Could you check a few things on this model? Use its own coordinates, in mm. Face numbers are marked on the shaded views. A direction names the side the tool comes from. Give positions to 0.01 mm unless a question says otherwise; leave off trailing zeros. Loops run counter-clockwise (first coordinate to the right, second up) from the corner with the lowest first, then second, coordinate; pieces in that order, holes last. Notation, with made-up numbers: (81, 50.25) -> (117, 50.25) arc R33 cw to (117, 86.25) -> close; hole circle Ø9 at (38.25, 80.25). An arc over 180 degrees is marked (long way). Write each question's results on one line, items separated by ' | '. Start each with the question number.
Q1. If we section it at D-D, the plane z = 26.5: List the corners of the cut face in (x, y) for me.
Q2. Which directions (+Z, -Z, +X, -X, +Y, -Y) give clear straight access to the entire face, cutting with the end or side of a thin tool? Please do the marked faces 1 and 2.
Q3. If we section it at C-C, the plane y = 16: List the corners of the cut face in (x, z) for me.
Q4. We'd pull the mould along Y, two halves only. Please class the marked faces 3, 4 and 5: released by +Y, released by -Y, zero draft, split by the parting line, or undercut.
Q5. If I drill on line 1 along X through (y, z) = (52.2, 42); line 2 along Y through (x, z) = (-21.5, 39); line 3 along Z through (x, y) = (9, 43), over which ranges is the centre line in solid material (lowest first)?
Q6. If we section it at A-A, the plane y = 7.5: List the corners of the cut face in (x, z) for me.
Q7. If we section it at B-B, the plane z = 37: List the corners of the cut face in (x, y) for me, plus the area to 3 significant figures.
Q8. Will these pins go through, and if not, where does the flat tip stop? P1, Ø0.9, axis at x = 8.5, y = 39, coming from the +Z side; P2, Ø5, axis at y = 33, z = 8.5, coming from the -X side.
Autodesk Inventor part; units mm, degrees
ref_plane "YZ Plane" through (0, 0, 0) normal (1, 0, 0) x (0, 1, 0)
ref_plane "XZ Plane" through (0, 0, 0) normal (0, 1, 0) x (-1, 0, 0)
ref_plane "XY Plane" through (0, 0, 0) normal (0, 0, 1) x (1, 0, 0)
sketch "Szkic1" plane through (0, 0, 0) normal (0, 0, 1) x (1, 0, 0)
  line L0 (-24.1556, -3.6171) -> (-24.1556, -6.6171)
  line L1 (-24.1556, -6.6171) -> (10.8444, -6.6171)
  line L2 (10.8444, -6.6171) -> (10.8444, 53.3829)
  line L3 (7.8444, 50.3829) -> (7.8444, -3.6171)
  line L4 (7.8444, -3.6171) -> (-24.1556, -3.6171)
  line L5 (-24.1556, 53.3829) -> (-24.1556, 50.3829)
  line L6 (-24.1556, 50.3829) -> (7.8444, 50.3829)
  line L7 (-24.1556, 53.3829) -> (10.8444, 53.3829)
  point P0 (0, 0)
  dimension "d2" = 60
  dimension "d87" = 3
  dimension "d89" = 3
  dimension "d90" = 3
  dimension "d123" = 35
  dimension "d124" = 35
extrude "Wyciągnięcie proste1" add sketch "Szkic1" along normal blind 55.5
fillet "Zaokrąglenie1" radius 0.5 2 edges at (7.8444, -3.6171, 27.75) (7.8444, 50.3829, 27.75)
sketch "Szkic9" plane through (7.8444, -3.1171, 0) normal (-1, 0, 0) x (0, 0, 1)
  line L0 (42.5, 5.5) -> (0.5, 5.5)
  line L1 (0.5, 5.5) -> (0.5, 47.5)
  line L2 (0.5, 47.5) -> (42.5, 47.5)
  line L3 (42.5, 47.5) -> (42.5, 5.5)
  line L4 (0, 53) -> (55.5, 53)
  line L5 (0, 53) -> (0, 0)
  line L6 (55.5, 0) -> (0, 0)
  line L7 (55.5, 53) -> (55.5, 0)
  line L8 (37, 14) -> (37, 8) construction
  line L9 (35.5, 14) -> (35.5, 8)
  line L10 (38.5, 8) -> (38.5, 14)
  arc A0 (38.5, 14) -> (35.5, 14) centre (37, 14) ccw
  arc A1 (35.5, 8) -> (38.5, 8) centre (37, 8) ccw
  line L11 (37, 45) -> (37, 39) construction
  line L12 (35.5, 45) -> (35.5, 39)
  line L13 (38.5, 39) -> (38.5, 45)
  arc A2 (38.5, 45) -> (35.5, 45) centre (37, 45) ccw
  arc A3 (35.5, 39) -> (38.5, 39) centre (37, 39) ccw
  line L14 (6, 14) -> (6, 8) construction
  line L15 (4.5, 14) -> (4.5, 8)
  line L16 (7.5, 8) -> (7.5, 14)
  arc A4 (7.5, 14) -> (4.5, 14) centre (6, 14) ccw
  arc A5 (4.5, 8) -> (7.5, 8) centre (6, 8) ccw
  line L17 (6, 45) -> (6, 39) construction
  line L18 (4.5, 45) -> (4.5, 39)
  line L19 (7.5, 39) -> (7.5, 45)
  arc A6 (7.5, 45) -> (4.5, 45) centre (6, 45) ccw
  arc A7 (4.5, 39) -> (7.5, 39) centre (6, 39) ccw
  line L20 (21.5, 29.5) -> (21.5, 23.5) construction
  line L21 (10.5, 29.5) -> (10.5, 23.5)
  line L22 (32.5, 23.5) -> (32.5, 29.5)
  arc A8 (32.5, 29.5) -> (10.5, 29.5) centre (21.5, 29.5) ccw
  arc A9 (10.5, 23.5) -> (32.5, 23.5) centre (21.5, 23.5) ccw
  point P0 (0, 3.1171)
  point P1 (37, 11)
  point P2 (6, 11)
  point P3 (37, 42)
  point P4 (6, 42)
  point P5 (21.5, 26.5)
  dimension "d128" = 42
  dimension "d129" = 42
  dimension "d130" = 5.5
  dimension "d131" = 0.5
  dimension "d132" = 53
  dimension "d133" = 5.5
  dimension "d134" = 5.5
  dimension "d135" = 5.5
  dimension "d136" = 5.5
  dimension "d137" = 5.5
  dimension "d138" = 5.5
  dimension "d139" = 5.5
  dimension "d140" = 5.5
  dimension "d141" = 21
  dimension "d142" = 21
  dimension "d143" = 3
  dimension "d144" = 3
  dimension "d145" = 3
  dimension "d146" = 3
  dimension "d147" = 3
  dimension "d148" = 3
  dimension "d149" = 3
  dimension "d150" = 3
  dimension "d151" = 3
  dimension "d152" = 22
extrude "Wyciągnięcie proste4" cut sketch "Szkic9" against normal blind 3 contours A0 L10 A1 L9 | A2 L13 A3 L12 | A4 L16 A5 L15 | A6 L19 A7 L18 | A8 L22 A9 L21
sketch "Szkic10" plane through (-24.1556, -6.6171, 0) normal (0, -1, 0) x (1, 0, 0)
  line L0 (0, 0) -> (35, 0)
  line L1 (35, 0) -> (35, 55.5)
  line L2 (0, 55.5) -> (35, 55.5)
  line L3 (0, 0) -> (0, 55.5)
  line L4 (32, 55.5) -> (32, 0)
  line L5 (0, 28.5) -> (32, 28.5)
  line L6 (32, 10.5) -> (32, 32.5)
  line L7 (0, 28.5) -> (32, 0)
  point P0 (24.1556, 0)
  dimension "d155" = 28.5
extrude "Wyciągnięcie proste5" cut sketch "Szkic10" against normal up to surface (60 mm away) contours L3 L7 L0
sketch "Szkic11" plane through (-24.1556, -6.6171, 55.5) normal (0, -1, 0) x (1, 0, 0)
  line L0 (0, -27) -> (32, -55.5)
  line L1 (32, -55.5) -> (35, -55.5)
  line L2 (35, -55.5) -> (35, 0)
  line L3 (0, 0) -> (35, 0)
  line L4 (0, -27) -> (0, 0)
  line L5 (31.5, -55.0547) -> (31.5, 0)
  line L6 (32, 0) -> (32, -55.5)
  point P0 (24.1556, -55.5)
  point P1 (7.75, -13.5)
  point P2 (23.75, -13.5)
  dimension "d158" = 13.5
  dimension "d159" = 13.5
  dimension "d160" = 16
  dimension "d161" = 31.5
  dimension "d162" = 7.75
hole "Otwór7" at (-16.4056, -6.6171, 42) at (-0.4056, -6.6171, 42) direction (0, 1, 0) diameter 5 end through all
chamfer "Faza5" distance 4 angle 45 2 edges at (-24.1556, -5.1171, 55.5) (-24.1556, 51.8829, 55.5)
fillet "Zaokrąglenie6" radius 3 6 edges at (-24.1556, -5.1171, 28.5) (-24.1556, 51.8829, 28.5) (-24.1556, 51.8829, 51.5) (-20.1556, 51.8829, 55.5) (-24.1556, -5.1171, 51.5) (-20.1556, -5.1171, 55.5)
sketch "Szkic12" plane through (10.8444, -6.6171, 0) normal (1, 0, 0) x (0, 0, -1)
  line L0 (-55.5, 57) -> (-0.4453, 57)
  arc A0 (-7.5, 42.5) -> (-4.5, 42.5) centre (-6, 42.5) ccw
  line L1 (-7.5, 42.5) -> (-7.5, 48.5)
  arc A1 (-4.5, 48.5) -> (-7.5, 48.5) centre (-6, 48.5) ccw
  line L2 (-4.5, 48.5) -> (-4.5, 42.5)
  arc A2 (-38.5, 42.5) -> (-35.5, 42.5) centre (-37, 42.5) ccw
  line L3 (-38.5, 42.5) -> (-38.5, 48.5)
  arc A3 (-35.5, 48.5) -> (-38.5, 48.5) centre (-37, 48.5) ccw
  line L4 (-35.5, 48.5) -> (-35.5, 42.5)
  arc A4 (-38.5, 11.5) -> (-35.5, 11.5) centre (-37, 11.5) ccw
  line L5 (-38.5, 11.5) -> (-38.5, 17.5)
  arc A5 (-35.5, 17.5) -> (-38.5, 17.5) centre (-37, 17.5) ccw
  line L6 (-35.5, 17.5) -> (-35.5, 11.5)
  arc A6 (-7.5, 11.5) -> (-4.5, 11.5) centre (-6, 11.5) ccw
  line L7 (-7.5, 11.5) -> (-7.5, 17.5)
  arc A7 (-4.5, 17.5) -> (-7.5, 17.5) centre (-6, 17.5) ccw
  line L8 (-4.5, 17.5) -> (-4.5, 11.5)
  arc A8 (-32.5, 27) -> (-10.5, 27) centre (-21.5, 27) ccw
  line L9 (-32.5, 27) -> (-32.5, 33)
  arc A9 (-10.5, 33) -> (-32.5, 33) centre (-21.5, 33) ccw
  line L10 (-10.5, 33) -> (-10.5, 27)
  line L11 (0, 0) -> (0, 60)
  line L12 (0, 60) -> (-55.5, 60)
  line L13 (-55.5, 0) -> (-55.5, 60)
  line L14 (0, 0) -> (-55.5, 0)
  line L15 (-0.4453, 3) -> (-55.5, 3)
  line L16 (-55.5, 57) -> (-45.5, 57)
  line L17 (-45.5, 57) -> (-45.5, 37)
  line L18 (-45.5, 37) -> (-55.5, 37)
  line L19 (-55.5, 37) -> (-55.5, 57)
  point P0 (0, 6.6171)
  dimension "d174" = 20
  dimension "d175" = 10
extrude "Wyciągnięcie proste6" cut sketch "Szkic12" against normal through all contours L0 L17 L18 L13
fillet "Zaokrąglenie7" radius 3 3 edges at (9.0944, 50.3829, 45.5) (9.3444, 30.3829, 45.5) (9.3444, 30.3829, 55.5)
equation "\"d124\" = d123"
equation "\"d130\" = -0.5 * d129 + 0.5 * d132"
properties part number "CNCM_ALU_Y_Axis_Nema_17_Mount"
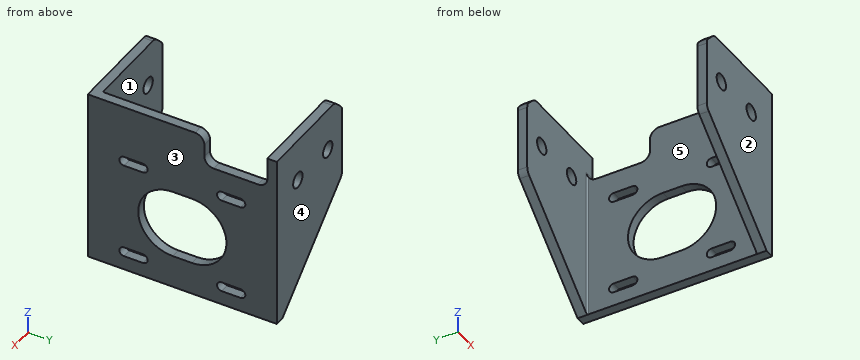
Final values:
1) outline: (-21.91, -6.62) -> (10.84, -6.62) -> (10.84, 10.58) -> (7.84, 10.58) -> (7.84, -3.12) arc R0.5 cw to (7.34, -3.62) -> (-21.91, -3.62) -> close; (-21.91, 50.38) -> (7.34, 50.38) arc R0.5 cw to (7.84, 49.88) -> (7.84, 36.18) -> (10.84, 36.18) -> (10.84, 53.38) -> (-21.91, 53.38) -> close
2) face 1: +Z, -Z, -X | face 2: +Z, -Z, +X, -X, -Y
3) outline: (7.84, 0) -> (10.84, 0) -> (10.84, 11.41) -> (7.84, 11.41) -> close; (7.84, 31.59) -> (10.84, 31.59) -> (10.84, 55.5) -> (7.84, 55.5) -> close
4) face 3: zero draft | face 4: released by +Y | face 5: undercut
5) line 1: x = -24.16 to -18.91, -13.91 to -2.91, 2.09 to 10.84 | line 2: y = -6.62 to -3.62, 50.38 to 53.38 | line 3: z = 0 to 5, 7 to 36, 38 to 45.5
6) outline: (7.84, 0) -> (10.84, 0) -> (10.84, 4.5) -> (7.84, 4.5) -> close; (7.84, 7.5) -> (10.84, 7.5) -> (10.84, 35.5) -> (7.84, 35.5) -> close; (7.84, 38.5) -> (10.84, 38.5) -> (10.84, 55.5) -> (7.84, 55.5) -> close
7) outline: (-24.16, -6.62) -> (10.84, -6.62) -> (10.84, 3.38) -> (7.84, 3.38) -> (7.84, -3.12) arc R0.5 cw to (7.34, -3.62) -> (-24.16, -3.62) -> close; (-24.16, 50.38) -> (7.34, 50.38) arc R0.5 cw to (7.84, 49.88) -> (7.84, 43.38) -> (10.84, 43.38) -> (10.84, 53.38) -> (-24.16, 53.38) -> close; (7.84, 12.38) -> (10.84, 12.38) -> (10.84, 34.38) -> (7.84, 34.38) -> close | area: 318 mm²
8) P1: stops at z = 45.5 | P2: stops at x = 7.84
